Here's how the part is built. I have some questions about the finished solid (model axes, mm). Face numbers are marked on the shaded views. A direction names the side the tool comes from. Coordinates: 2 decimals unless noted, no trailing zeros. Write each loop counter-clockwise with the first axis right and the second up, starting at its lowest first coordinate (ties: lowest second). Pieces come first, ordered by that corner, then holes. Notation, with made-up numbers: (32.5, -17) -> (72.5, -17) arc R13 ccw to (72.5, 7) -> close; hole circle Ø1 at (59, 68). An arc over 180 degrees is marked (long way). Use a Markdown table: item, result. Add a question column.
Item 1: Imagine slicing it at C-C, the plane z = -1.5. Write out the boundary of the cut face in (x, y).
Item 2: Will these pins go through, and if not, where does the flat tip stop? pin 1 Ø1.8 at (x, z) = (-28.45, 0) entering from +Y; pin 2 Ø2 at (x, y) = (19.5, 4.5) entering from +Z; pin 3 Ø1 at (x, y) = (-16.5, 3.5) entering from -Z.
Item 3: Imagine slicing it at B-B, the plane x = -25.3. Write out the boundary of the cut face in (y, z).
Item 4: Imagine slicing it at D-D, the plane y = 7. Write out the boundary of the cut face in (x, z), and give its area (3 significant figures).
Item 5: If I drill on line 1 along Y through (x, z) = (21.5, 3.25); line 2 along Z through (x, y) = (19, 2.25); line 3 along Z through (x, y) = (-18.5, 3.25), over which ranges is the centre line in solid material (lowest first)? Write a range as from..to.
Item 6: On a 3-axis mill with a long thin cutter (end or side, diameter ignored), from which of +Z, -Z, +X, -X, +Y, -Y can I reach the whole of each face in a straight line? I mean the marked faces 1 and 2. Say none if no direction works.
Item 7: Imagine slicing it at A-A, the plane y = 3. Count the separate pieces of the cut face and the enclosed holes in it, and give its area (3 significant figures).
```python
from build123d import *

# Parameters (mm, degrees)
SKETCH1_R           = 0.7
BOSS_EXTRUDE1_DEPTH = 3.85
FILLET1_R           = 10
SKETCH2_R           = 4.9
BOSS_EXTRUDE2_DEPTH = 4.1


with BuildPart() as part:
    # Sketch1 → Boss-Extrude1 (new body)
    with BuildSketch(Plane(origin=(0, 0, 0), x_dir=(1, 0, 0), z_dir=(0, 1, 0))):
        with BuildLine():
            Line((27.613034708, 3.983491659), (0, 6.5))
            Line((0, 6.5), (-27.613034708, 3.983491659))
            ThreePointArc((-27.613034708, 3.983491659), (-31.25, 0), (-27.613034708, -3.983491659))
            Line((-27.613034708, -3.983491659), (0, -6.5))
            Line((0, -6.5), (27.613034708, -3.983491659))
            ThreePointArc((27.613034708, -3.983491659), (31.25, 0), (27.613034708, 3.983491659))
        make_face()
        with Locations(Location((28.45, 0, 0), (0, 0, 90))):
            Circle(SKETCH1_R, mode=Mode.SUBTRACT)
        with Locations(Location((25.3, 0, 0), (0, 0, 90))):
            Circle(SKETCH1_R, mode=Mode.SUBTRACT)
        with Locations(Location((22.15, 0, 0), (0, 0, 90))):
            Circle(SKETCH1_R, mode=Mode.SUBTRACT)
        with Locations(Location((19, 0, 0), (0, 0, 90))):
            Circle(SKETCH1_R, mode=Mode.SUBTRACT)
        with Locations(Location((15.85, 0, 0), (0, 0, 90))):
            Circle(SKETCH1_R, mode=Mode.SUBTRACT)
        with Locations(Location((-15.85, 0, 0), (0, 0, 90))):
            Circle(SKETCH1_R, mode=Mode.SUBTRACT)
        with Locations(Location((-19, 0, 0), (0, 0, 90))):
            Circle(SKETCH1_R, mode=Mode.SUBTRACT)
        with Locations(Location((-22.15, 0, 0), (0, 0, 90))):
            Circle(SKETCH1_R, mode=Mode.SUBTRACT)
        with Locations(Location((-25.3, 0, 0), (0, 0, 90))):
            Circle(SKETCH1_R, mode=Mode.SUBTRACT)
        with Locations(Location((-28.45, 0, 0), (0, 0, 90))):
            Circle(SKETCH1_R, mode=Mode.SUBTRACT)
    extrude(amount=BOSS_EXTRUDE1_DEPTH)

    # Fillet1
    fillet1_edges = [part.edges().sort_by_distance(p)[0] for p in [
        (0, 1.925, 6.5),
        (0, 1.925, -6.5),
    ]]
    fillet(fillet1_edges, radius=FILLET1_R)

    # Sketch2 → Boss-Extrude2 (add)
    with BuildSketch(Plane(origin=(0, 3.85, 0), x_dir=(1, 0, 0), z_dir=(0, 1, 0))):
        with Locations(Location((0, 0, 0), (0, 0, 270))):
            Circle(SKETCH2_R)
    extrude(amount=BOSS_EXTRUDE2_DEPTH)


solid = part.part
```
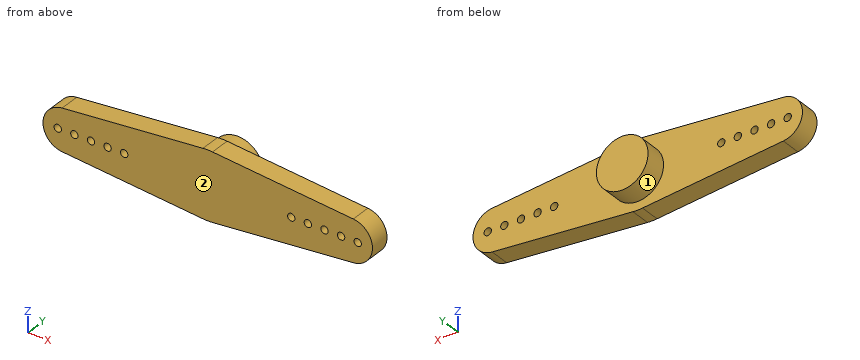
Ans:
| question | item | result |
|---|---|---|
| 1 | outline | (-30.96, 0) -> (30.96, 0) -> (30.96, 3.85) -> (4.66, 3.85) -> (4.66, 7.95) -> (-4.66, 7.95) -> (-4.66, 3.85) -> (-30.96, 3.85) -> close |
| 2 | pin 1 | stops at y = 3.85 |
| 2 | pin 2 | stops at z = 4.79 |
| 2 | pin 3 | stops at z = -5.04 |
| 3 | outline | (0, -4.19) -> (3.85, -4.19) -> (3.85, -0.7) -> (0, -0.7) -> close; (0, 0.7) -> (3.85, 0.7) -> (3.85, 4.19) -> (0, 4.19) -> close |
| 4 | outline | circle Ø9.8 at (0, 0) |
| 4 | area | 75.4 mm^2 |
| 5 | line 1 | y = 0..3.85 |
| 5 | line 2 | z = -4.77..-0.7, 0.7..4.77 |
| 5 | line 3 | z = -4.81..-0.49, 0.49..4.81 |
| 6 | face 1 | +Y |
| 6 | face 2 | +Z, -Z, +X, -X, -Y |
| 7 | separate pieces | 1 |
| 7 | enclosed holes | 10 |
| 7 | area | 608 mm^2 |
